```python
from build123d import *

# Parameters (mm, degrees)
BASE_FLANGE1_DEPTH           = 3
SKETCH7_R                    = 8
SKETCH7_R_2                  = 2
CUT_EXTRUDE1_DEPTH           = 3
EDGE_FLANGE1_START           = -27.5
EDGE_FLANGE1_DEPTH           = 55
EDGE_FLANGE1_START_2         = -28.7366
EDGE_FLANGE1_2_DEPTH         = 1.2366
EDGE_FLANGE1_3_DEPTH         = 55
EDGE_FLANGE2_STRIP_W         = 13.4732
EDGE_FLANGE2_STRIP_H         = 3
EDGE_FLANGE2_STRIP_CUT_DEPTH = 55
EDGE_FLANGE2_DEPTH           = 55
BOSS_EXTRUDE1_DEPTH          = 3
SKETCH18_R                   = 8
SKETCH18_R_2                 = 1.5
CUT_EXTRUDE2_DEPTH           = 3
SKETCH19_W                   = 24
SKETCH19_H                   = 8.5
CUT_EXTRUDE3_DEPTH           = 72


# Read off the part's stored shape, not the designer's step: Edge-Flange1
# Sheet-metal steps are written as plain solids
with BuildPart() as part:
    # Sketch1 → Base-Flange1 (new body)
    with BuildSketch(Plane(origin=(0, 0, 0), x_dir=(1, 0, 0), z_dir=(0, 1, 0))):
        Polygon((-37.5, 21), (-37.5, -21), (-27.5, -31), (-27.5, -35), (27.5, -35), (27.5, 35), (-27.5, 35), (-27.5, 31), align=None)
    extrude(amount=-BASE_FLANGE1_DEPTH)

    # Sketch7 → Cut-Extrude1 (cut)
    with BuildSketch(Plane(origin=(0, 0, 0), x_dir=(1, 0, 0), z_dir=(0, 1, 0))):
        with Locations(Location((-7.5, 0, 0), (0, 0, 270))):
            Circle(SKETCH7_R)
        with Locations(Location((-18, 10.5, 0), (0, 0, 270))):
            Circle(SKETCH7_R_2)
        with Locations(Location((3, 10.5, 0), (0, 0, 270))):
            Circle(SKETCH7_R_2)
        with Locations(Location((3, -10.5, 0), (0, 0, 270))):
            Circle(SKETCH7_R_2)
        with Locations(Location((-18, -10.5, 0), (0, 0, 270))):
            Circle(SKETCH7_R_2)
    extrude(amount=-CUT_EXTRUDE1_DEPTH, mode=Mode.SUBTRACT)

    # Edge-Flange1 outline → Edge-Flange1 (cut)
    with BuildSketch(Plane.YZ.offset(EDGE_FLANGE1_START)):
        with BuildLine():
            Line((-3, 35), (-3, 31.2634))
            ThreePointArc((-3, 31.2634), (-2.154295979, 33.630867001), (0, 34.926677222))
            Line((0, 34.926677222), (0, 35))
            Line((0, 35), (-3, 35))
        make_face()
        with BuildLine():
            ThreePointArc((0, -34.926677222), (-2.154295979, -33.630867001), (-3, -31.2634))
            Line((-3, -31.2634), (-3, -35))
            Line((-3, -35), (0, -35))
            Line((0, -35), (0, -34.926677222))
        make_face()
    extrude(amount=EDGE_FLANGE1_DEPTH, mode=Mode.SUBTRACT)

    # Edge-Flange1 2 outline → Edge-Flange1 2 (cut)
    with BuildSketch(Plane.YZ.offset(EDGE_FLANGE1_START_2)):
        with BuildLine():
            Line((-3, 29.7634), (0, 29.7634))
            Line((0, 29.7634), (0, 34.926677222))
            ThreePointArc((0, 34.926677222), (-2.154295979, 33.630867001), (-3, 31.2634))
            Line((-3, 31.2634), (-3, 29.7634))
        make_face()
        with BuildLine():
            Line((0, -34.926677222), (0, -29.7634))
            Line((0, -29.7634), (-3, -29.7634))
            Line((-3, -29.7634), (-3, -31.2634))
            ThreePointArc((-3, -31.2634), (-2.154295979, -33.630867001), (0, -34.926677222))
        make_face()
    extrude(amount=EDGE_FLANGE1_2_DEPTH, mode=Mode.SUBTRACT)

    # Edge-Flange1 3 outline → Edge-Flange1 3 (add)
    with BuildSketch(Plane.YZ.offset(EDGE_FLANGE1_START)):
        with BuildLine():
            Line((0, 34.926677222), (0, 31.2634))
            ThreePointArc((0, 31.2634), (0.215745145, 31.784254855), (0.7366, 32))
            Line((0.7366, 32), (69, 32))
            Line((69, 32), (69, 35))
            Line((69, 35), (0.7366, 35))
            ThreePointArc((0.7366, 35), (0.36647982, 34.981624121), (0, 34.926677222))
        make_face()
        with BuildLine():
            ThreePointArc((0.7366, -32), (0.215745145, -31.784254855), (0, -31.2634))
            Line((0, -31.2634), (0, -34.926677222))
            ThreePointArc((0, -34.926677222), (0.36647982, -34.981624121), (0.7366, -35))
            Line((0.7366, -35), (69, -35))
            Line((69, -35), (69, -32))
            Line((69, -32), (0.7366, -32))
        make_face()
    extrude(amount=EDGE_FLANGE1_3_DEPTH)

    # Edge-Flange2 strip (across the edge) → Edge-Flange2 strip cut (cut)
    with BuildSketch(Plane(origin=(-27.5, 69, 32), x_dir=(0, -1, 0), z_dir=(1, 0, 0))):
        with Locations((-3, -1.5)):
            Rectangle(EDGE_FLANGE2_STRIP_W, EDGE_FLANGE2_STRIP_H)
    extrude(amount=EDGE_FLANGE2_STRIP_CUT_DEPTH, mode=Mode.SUBTRACT)

    # Edge-Flange2 section (across the edge) → Edge-Flange2 (add)
    with BuildSketch(Plane(origin=(-27.5, 69, 32), x_dir=(0, -1, 0), z_dir=(1, 0, 0))):
        with BuildLine():
            Line((0, 0.7366), (0, 63.99))
            Line((0, 63.99), (3, 63.99))
            Line((3, 63.99), (3, 0.7366))
            ThreePointArc((3, 0.7366), (3.215745145, 0.215745145), (3.7366, 0))
            Line((3.7366, 0), (3.7366, -3))
            ThreePointArc((3.7366, -3), (1.094424801, -1.905575199), (0, 0.7366))
        make_face()
    extrude(amount=EDGE_FLANGE2_DEPTH)

    # Sketch17 → Boss-Extrude1 (add)
    with BuildSketch(Plane(origin=(0, 69, 0), x_dir=(1, 0, 0), z_dir=(0, 1, 0))):
        Polygon((-27.5, -29.7634), (-28.7366, -29.7634), (-37.5, -21), (-37.5, 21), (-28.7366, 29.7634), (-27.5, 29.7634), align=None)
    extrude(amount=-BOSS_EXTRUDE1_DEPTH)

    # Sketch18 → Cut-Extrude2 (cut)
    with BuildSketch(Plane(origin=(0, 69, 0), x_dir=(1, 0, 0), z_dir=(0, 1, 0))):
        with Locations(Location((-7.5, 0, 0), (0, 0, 270))):
            Circle(SKETCH18_R)
        with Locations(Location((-7.5, 23, 0), (0, 0, 270))):
            Circle(SKETCH18_R_2)
        with Locations(Location((-7.5, -23, 0), (0, 0, 270))):
            Circle(SKETCH18_R_2)
    extrude(amount=-CUT_EXTRUDE2_DEPTH, mode=Mode.SUBTRACT)

    # Sketch19 → Cut-Extrude3 (cut)
    with BuildSketch(Plane(origin=(0, 69, 0), x_dir=(1, 0, 0), z_dir=(0, 1, 0))):
        with Locations((-25.5, 0)):
            Rectangle(SKETCH19_W, SKETCH19_H)
    extrude(amount=-CUT_EXTRUDE3_DEPTH, mode=Mode.SUBTRACT)


solid = part.part
```
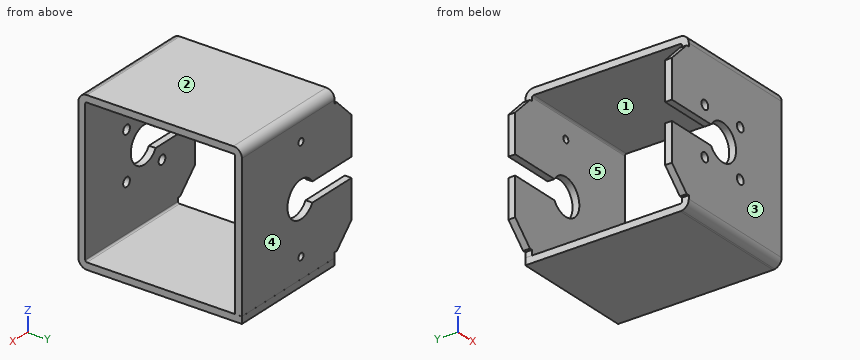
Could you check a few things on this model? Use its own coordinates, in mm. Face numbers are marked on the shaded views. A direction names the side the tool comes from. Coordinates: 2 decimals unless noted, no trailing zeros. Order: outer loops, then holes, each group sorted by start corner. A loop starts at its lowest first (then second) coordinate and runs counter-clockwise, first axis right, second up. Notation, with made-up numbers: M 64,-21.5 L 115,-21.5 A8 ccw 115,-8.5 Z; hole C 49,35.5 d1. An arc over 180 degrees is marked long. Use one line per item in the form item = value. Start each with the question number.
1. Suppose I cut it at B-B on y = 11. Write out the boundary of the cut face in (x, z).
2. Suppose I cut it at C-C on x = -30. Write out the boundary of the cut face in (y, z), then the cut area to 3 significant figures.
3. On a 3-axis mill with a long thin cutter (end or side, diameter ignored), from which of +Z, -Z, +X, -X, +Y, -Y can I reach the whole of each face in a straight line? I mean the marked faces 4 and 5. Say none if no direction works.
4. We'd pull the mould along Y, two halves only. Please class the marked faces 1, 2 and 3: +Y half, -Y half, draft (parallel to the pull), parting line (faces both ways), or undercut.
5. For pin 1 (1.5 mm diameter, centred on x = -25.5, y = -1.5, fed in from +Z); pin 2 (2.5 mm diameter, centred on x = -29, y = 67.5, fed in from -Z); pin 3 (6 mm diameter, centred on y = 48.5, z = -33, fed in from -X); pin 4 (10 mm diameter, centred on y = 47, z = 25.5, fed in from +X), each with a flat end and sliding along its axis, tell me the tip position at first contact or that it passes through.
6. Please list where these lines run through material, in increasing order: line 1 (X direction, y = -1.65, z = -10.5); line 2 (Y direction, x = -25.5, z = -17.5); line 3 (Z direction, x = 6, y = 49.5).
7. Suppose I cut it at A-A on z = -25.5. Write out the boundary of the cut face in (x, y), then the cut area to 3 significant figures.
8. Suppose I cut it at D-D on z = -10.5. Write out the boundary of the cut face in (x, y), then the cut area to 3 significant figures.
Geometry says:
q1.outline = M -27.5,-35 L 27.5,-35 L 27.5,-32 L -27.5,-32 Z; M -27.5,32 L 27.5,32 L 27.5,35 L -27.5,35 Z
q2.outline = M -3,-28.5 L 0,-28.5 L 0,-4.25 L -3,-4.25 Z; M -3,4.25 L 0,4.25 L 0,28.5 L -3,28.5 Z; M 66,-28.5 L 69,-28.5 L 69,-4.25 L 66,-4.25 Z; M 66,4.25 L 69,4.25 L 69,28.5 L 66,28.5 Z
q2.area = 291 mm^2
q3.face_4 = +Z, -Z, +X, -X, +Y
q3.face_5 = +X, -X
q4.face_1 = undercut
q4.face_2 = draft
q4.face_3 = -Y half
q5.pin_1 = 34.69
q5.pin_2 = -29.76
q5.pin_3 = -27.5
q5.pin_4 = through
q6.line_1 = -37.5 to -20, -16 to 1, 5 to 27.5
q6.line_2 = -3 to 0, 66 to 69
q6.line_3 = -35 to -32, 32 to 35
q7.outline = M -33,-3 L 27.5,-3 L 27.5,0 L -33,0 Z; M -33,66 L 27.5,66 L 27.5,69 L -33,69 Z
q7.area = 363 mm^2
q8.outline = M -37.5,-3 L -20,-3 L -20,0 L -37.5,0 Z; M -37.5,66 L 27.5,66 L 27.5,69 L -37.5,69 Z; M -16,-3 L 1,-3 L 1,0 L -16,0 Z; M 5,-3 L 27.5,-3 L 27.5,0 L 5,0 Z
q8.area = 366 mm^2
